Design review of the part shown in the three views and the two pictorial views. Dimensions are in mm from the part's minimum x, y and z. A direction names the side the tool comes from. Give positions to 0.01 mm unless a question says otherwise; leave off trailing zeros. Order: outer loops, then holes, each group sorted by start corner. A loop starts at its lowest first (then second) coordinate and runs counter-clockwise, first axis right, second up.
Item 1: Machinability: for the marked faces 1, 2 and 3, which of the approach directions +Z, -Z, +X, -X, +Y, -Y give a long, thin tool a straight path to every point of the face, cutting with its end or side? Answer none if there is none.
Item 2: Consider section D-D (y = 4). Give the boundary of the cut face in (x, z).
Item 3: Consider section B-B (y = 10). Give the boundary of the cut face in (x, z) (1 decimal).
Item 4: Consider section A-A (x = 7). Give the boundary of the cut face in (y, z) (1 decimal), plus the area to 3 significant figures.
Item 5: For probe 1 along Z at (x, y) = (97.5, 3); probe 2 along X at (y, z) = (5.5, 48.5); probe 3 along Z at (x, y) = (90, 6.75), list the stretches that pass through material, from the lowest coordinate up.
Item 6: Consider section C-C (z = 21). Give the boundary of the cut face in (x, y).
Item 7: For P1, Ø6.5, axis at y = 8, z = 29.5, coming from the +X side; P2, Ø3, axis at x = 32.5, y = 1.5, coming from the -Z side; P3, Ø4, axis at y = 7, z = 39, coming from the -X side, all flat-tipped, find the tip position at first contact; note any pin that passes through.
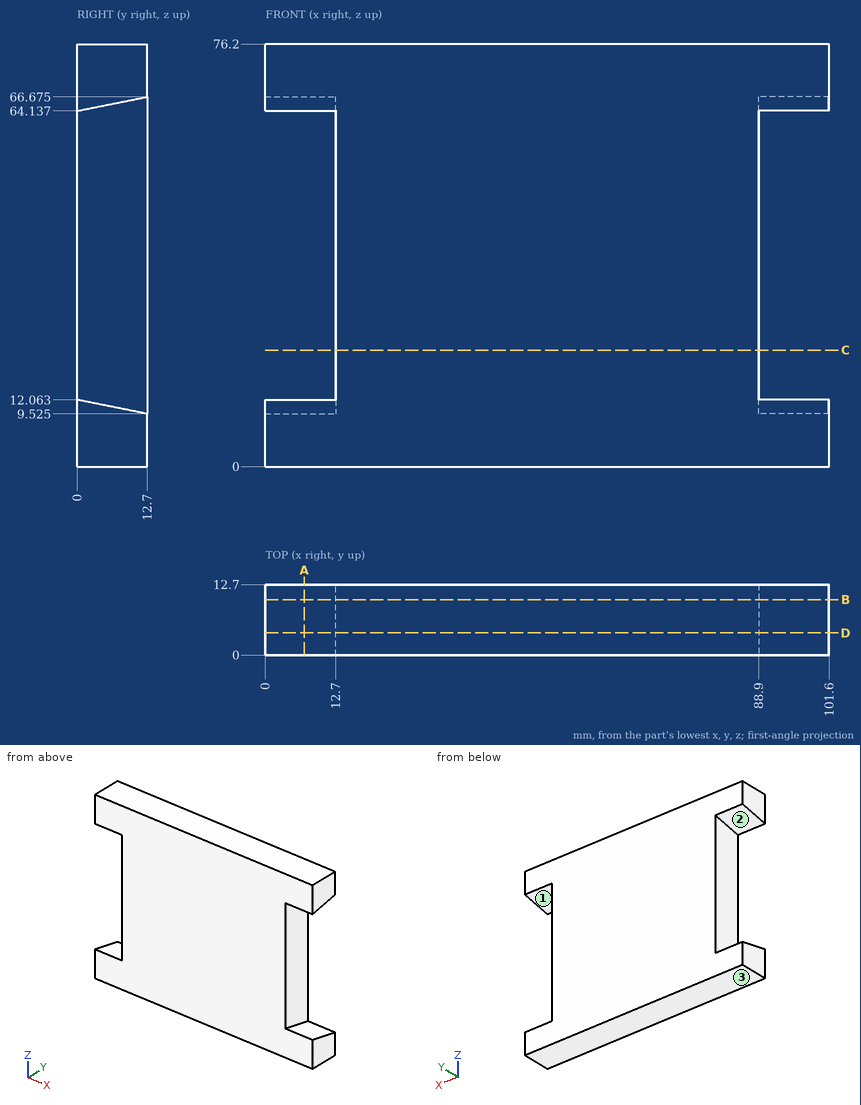
Resolved:
1. face 1: +X, +Y
1. face 2: -X, +Y
1. face 3: -Z, +X, -X, +Y, -Y
2. outline: (0, 0) - (101.6, 0) - (101.6, 11.26) - (88.9, 11.26) - (88.9, 64.94) - (101.6, 64.94) - (101.6, 76.2) - (0, 76.2) - (0, 64.94) - (12.7, 64.94) - (12.7, 11.26) - (0, 11.26) - close
3. outline: (0, 0) - (101.6, 0) - (101.6, 10.1) - (88.9, 10.1) - (88.9, 66.1) - (101.6, 66.1) - (101.6, 76.2) - (0, 76.2) - (0, 66.1) - (12.7, 66.1) - (12.7, 10.1) - (0, 10.1) - close
4. outline: (0, 0) - (12.7, 0) - (12.7, 9.5) - (0, 12.1) - close; (0, 64.1) - (12.7, 66.7) - (12.7, 76.2) - (0, 76.2) - close
4. area: 274 mm2
5. probe 1: z = 0 to 11.46, 64.74 to 76.2
5. probe 2: x = 12.7 to 88.9
5. probe 3: z = 0 to 10.71, 65.49 to 76.2
6. outline: (12.7, 0) - (88.9, 0) - (88.9, 12.7) - (12.7, 12.7) - close
7. P1: stops at x = 88.9
7. P2: stops at z = 0
7. P3: stops at x = 12.7
